from build123d import *

# Parameters (mm, degrees)
SKETCH1_W           = 43
SKETCH1_H           = 21.2
SKETCH1_R           = 1.6
BOSS_EXTRUDE1_DEPTH = 1.3
SKETCH2_R           = 2
BOSS_EXTRUDE2_DEPTH = 15.5
FILLET1_R           = 1.5
SKETCH3_W           = 18.2
SKETCH3_H           = 17.3
BOSS_EXTRUDE3_DEPTH = 13.2


with BuildPart() as part:
    # Sketch1 → Boss-Extrude1 (new body)
    with BuildSketch(Plane.XY):
        with Locations((21.5, 10.6)):
            Rectangle(SKETCH1_W, SKETCH1_H)
        with Locations((21.5, 15.3)):
            Circle(SKETCH1_R, mode=Mode.SUBTRACT)
    extrude(amount=BOSS_EXTRUDE1_DEPTH)

    # Sketch2 → Boss-Extrude2 (add)
    with BuildSketch(Plane.XY.offset(1.3)):
        with Locations(Location((17.75, 15.9, 0), (0, 0, 180))):
            Circle(SKETCH2_R)
    extrude(amount=BOSS_EXTRUDE2_DEPTH)

    # Fillet1
    fillet1_edges = [part.edges().sort_by_distance(p)[0] for p in [
        (19.75, 15.9, 16.8),
    ]]
    fillet(fillet1_edges, radius=FILLET1_R)

    # Sketch3 → Boss-Extrude3 (add)
    with BuildSketch(Plane.XY.offset(1.3)):
        with Locations((36.5, 10.6)):
            Rectangle(SKETCH3_W, SKETCH3_H)
        with Locations((6.5, 10.6)):
            Rectangle(SKETCH3_W, SKETCH3_H)
    extrude(amount=BOSS_EXTRUDE3_DEPTH)


solid = part.part
The listing builds one solid part. Answer for the finished solid, in the listing's coordinates (mm). A direction names the side the tool comes from. Coordinates: 2 decimals unless noted, no trailing zeros. Write each loop counter-clockwise with the first axis right and the second up, starting at its lowest first coordinate (ties: lowest second). Pieces come first, ordered by that corner, then holes. Notation, with made-up numbers: M 83,-28 L 96,-28 A25 ccw 96,-4 Z; hole C 21,56 d6. An arc over 180 degrees is marked long. Put each result on its own line as item: value. Start each with the question number.
1. A cutting plane is placed at A-A on x = 21.5. Write down the section's boundary in (y, z), then the cut area to 3 significant figures.
2. For a pull along X with two mould halves and no side action, classify faces 1 (the cylindrical face through (19.748, 15.812, 8.202)), 2 (the flat face through (-2.6, 10, 8)), 3 (the flat face through (21, 11, 1.3)), 4 (the flat face through (18, 16, 16.8)) as pulls with the +X half, pulls with the -X half, needs draft (parallel to the pull), parting line crosses it, or undercut.
3. A cutting plane is placed at D-D on x = 37.5. Write down the section's boundary in (y, z).
4. A cutting plane is placed at C-C on y = 9.25. Write down the section's boundary in (x, z).
5. Flat-ended cylindrical pins translate along their axes: P1, Ø2, axis at x = -1.5, y = 7, coming from the -Z side; P2, Ø1.5, axis at x = 31, z = 12.5, coming from the -Y side; P3, Ø1.5, axis at x = 17, y = 11, coming from the +Z side. Find the tip coordinate at first contact, or state that the pin passes through.
6. A cutting plane is placed at B-B on z = 13.5. Write down the section's boundary in (x, y).
7. Which of the six approach directions +Z, -Z, +X, -X, +Y, -Y give full straight-line access (tool end or side, diameter ignored) to faces 5 (the flat face through (0, 10, 1)), 6 (the flat face through (6, 1.95, 8)), 7 (the flat face through (44, 11, 1.3)), 8 (the flat face through (6, 11, 14.5)), 9 (the flat face through (36, 11, 14.5))?
8. Consider line 1 (X direction, y = 18, z = 6.75); line 2 (Y direction, x = 21.5, z = 0.7); line 3 (X direction, y = 17, z = 11.75). Determine where each line is inside the solid, lowest interval first. Write a range as from..to.
Resolved:
1. outline: M 0,0 L 13.7,0 L 13.7,1.3 L 0,1.3 Z; M 16.9,0 L 21.2,0 L 21.2,1.3 L 16.9,1.3 Z
1. area: 23.4 mm2
2. face 1: undercut
2. face 2: pulls with the -X half
2. face 3: undercut
2. face 4: needs draft
3. outline: M 0,0 L 21.2,0 L 21.2,1.3 L 19.25,1.3 L 19.25,14.5 L 1.95,14.5 L 1.95,1.3 L 0,1.3 Z
4. outline: M -2.6,1.3 L 0,1.3 L 0,0 L 43,0 L 43,1.3 L 45.6,1.3 L 45.6,14.5 L 27.4,14.5 L 27.4,1.3 L 15.6,1.3 L 15.6,14.5 L -2.6,14.5 Z
5. P1: stops at z = 1.3
5. P2: stops at y = 1.95
5. P3: stops at z = 1.3
6. outline: M -2.6,1.95 L 15.6,1.95 L 15.6,19.25 L -2.6,19.25 Z; C 17.75,15.9 d4; M 27.4,1.95 L 45.6,1.95 L 45.6,19.25 L 27.4,19.25 Z
7. face 5: -Z, -X, +Y, -Y
7. face 6: +Z, +X, -X, -Y
7. face 7: -Z, +X, +Y, -Y
7. face 8: +Z, -X, +Y, -Y
7. face 9: +Z, +X, +Y, -Y
8. line 1: x = -2.6..15.6, 27.4..45.6
8. line 2: y = 0..13.7, 16.9..21.2
8. line 3: x = -2.6..15.6, 16.08..19.42, 27.4..45.6
